Geometry: final body of the model. Coordinates: model frame, mm. A direction names the side the tool comes from. Give positions to 0.01 mm unless a question says otherwise; leave off trailing zeros. Write each loop counter-clockwise with the first axis right and the second up, starting at its lowest first coordinate (ties: lowest second). Pieces come first, ordered by that corner, then holes.
```python
from build123d import *

# Parameters (mm, degrees)
SKETCH001_W   = 70
SKETCH001_H   = 30
SKETCH001_R   = 3.9
SKETCH001_W_2 = 16
SKETCH001_H_2 = 17
PAD001_DEPTH  = 5
SKETCH002_W   = 70
SKETCH002_H   = 30
PAD002_DEPTH  = 5
SKETCH003_W   = 120
SKETCH003_H   = 30
PAD003_DEPTH  = 5
SKETCH004_W   = 120
SKETCH004_H   = 30
PAD004_DEPTH  = 5
SKETCH005_W   = 5
SKETCH005_H   = 5
SKETCH005_R   = 1
PAD005_DEPTH  = 30
SKETCH007_W   = 5
SKETCH007_H   = 5
SKETCH007_R   = 1
PAD006_DEPTH  = 30
SKETCH008_W   = 5
SKETCH008_H   = 5
SKETCH008_R   = 1
PAD007_DEPTH  = 30
SKETCH009_W   = 5
SKETCH009_H   = 5
SKETCH009_R   = 1
PAD008_DEPTH  = 30
SKETCH_R      = 2.5
PAD_DEPTH     = 5


with BuildPart() as body001:
    # Sketch001 → Pad001 (new body)
    with BuildSketch(Plane.XZ):
        with Locations((0, 15)):
            Rectangle(SKETCH001_W, SKETCH001_H)
        with Locations((-20, 15)):
            Circle(SKETCH001_R, mode=Mode.SUBTRACT)
        with Locations((8, 8.5)):
            Rectangle(SKETCH001_W_2, SKETCH001_H_2, mode=Mode.SUBTRACT)
    extrude(amount=PAD001_DEPTH)


with BuildPart() as body001_1:
    # Body001 placement: moved
    add(body001.part.moved(Location((0, -60, 0))))


with BuildPart() as body002:
    # Sketch002 → Pad002 (new body)
    with BuildSketch(Plane.XZ):
        with Locations((-105, 15)):
            Rectangle(SKETCH002_W, SKETCH002_H)
    extrude(amount=PAD002_DEPTH)


with BuildPart() as body002_1:
    # Body002 placement: moved
    add(body002.part.moved(Location((105, 65, 0))))


with BuildPart() as body003:
    # Sketch003 → Pad003 (new body)
    with BuildSketch(Plane.YZ):
        with Locations((0, 15)):
            Rectangle(SKETCH003_W, SKETCH003_H)
    extrude(amount=PAD003_DEPTH)


with BuildPart() as body003_1:
    # Body003 placement: moved
    add(body003.part.moved(Location((30, 0, 0))))


with BuildPart() as body004:
    # Sketch004 → Pad004 (new body)
    with BuildSketch(Plane.YZ):
        with Locations((0, 15)):
            Rectangle(SKETCH004_W, SKETCH004_H)
    extrude(amount=PAD004_DEPTH)


with BuildPart() as body004_1:
    # Body004 placement: moved
    add(body004.part.moved(Location((-35, 0, 0))))


with BuildPart() as hole_in_the_right_frame:
    # Sketch005 → Pad005 (new body)
    with BuildSketch(Plane.XY):
        with Locations((27.5, 42.5)):
            Rectangle(SKETCH005_W, SKETCH005_H)
        with Locations((27.5, 42.5)):
            Circle(SKETCH005_R, mode=Mode.SUBTRACT)
    extrude(amount=PAD005_DEPTH)


with BuildPart() as hole_in_the_right_frame_1:
    # Body005 placement: moved
    add(hole_in_the_right_frame.part.moved(Location((0, 15, 0))))


with BuildPart() as hole_in_the_left_frame:
    # Sketch007 → Pad006 (new body)
    with BuildSketch(Plane.XY):
        with Locations((-27.5, 42.5)):
            Rectangle(SKETCH007_W, SKETCH007_H)
        with Locations((-27.5, 42.5)):
            Circle(SKETCH007_R, mode=Mode.SUBTRACT)
    extrude(amount=PAD006_DEPTH)


with BuildPart() as hole_in_the_left_frame_1:
    # Body006 placement: moved
    add(hole_in_the_left_frame.part.moved(Location((0, 15, 0))))


with BuildPart() as hole_in_the_left_frame1:
    # Sketch008 → Pad007 (new body)
    with BuildSketch(Plane.XY):
        with Locations((-27.5, -42.5)):
            Rectangle(SKETCH008_W, SKETCH008_H)
        with Locations((-27.5, -42.5)):
            Circle(SKETCH008_R, mode=Mode.SUBTRACT)
    extrude(amount=PAD007_DEPTH)


with BuildPart() as hole_in_the_left_frame1_1:
    # Body007 placement: moved
    add(hole_in_the_left_frame1.part.moved(Location((0, -15, 0))))


with BuildPart() as body008:
    # Sketch009 → Pad008 (new body)
    with BuildSketch(Plane.XY):
        with Locations((27.5, -42.5)):
            Rectangle(SKETCH009_W, SKETCH009_H)
        with Locations((27.5, -42.5)):
            Circle(SKETCH009_R, mode=Mode.SUBTRACT)
    extrude(amount=PAD008_DEPTH)


with BuildPart() as body008_1:
    # Body008 placement: moved
    add(body008.part.moved(Location((0, -15, 0))))


with BuildPart() as fusion:
    # Sketch → Pad (new body)
    with BuildSketch(Plane.XY):
        with BuildLine():
            Line((-35.022389, 65), (35, 65))
            ThreePointArc((45, 55), (42.071068, 62.071068), (35, 65))
            Line((45, 55), (45, -55))
            ThreePointArc((35, -65), (42.071068, -62.071068), (45, -55))
            Line((35, -65), (-35, -65))
            ThreePointArc((-45, -55), (-42.071068, -62.071068), (-35, -65))
            Line((-45, -55), (-45, 55.022389))
            ThreePointArc((-35.022389, 65), (-42.077625, 62.077625), (-45, 55.022389))
        make_face()
        with Locations((40, -55)):
            Circle(SKETCH_R, mode=Mode.SUBTRACT)
        with Locations((40, 55)):
            Circle(SKETCH_R, mode=Mode.SUBTRACT)
        with Locations((-40, -55)):
            Circle(SKETCH_R, mode=Mode.SUBTRACT)
        with Locations((-40, 55)):
            Circle(SKETCH_R, mode=Mode.SUBTRACT)
    extrude(amount=PAD_DEPTH)

    # Fusion: union Body001, Body002, Body003, Body004, Hole in the right frame, Hole in the left frame, Hole in the left frame1, Body008
    add(body001_1.part)
    add(body002_1.part)
    add(body003_1.part)
    add(body004_1.part)
    add(hole_in_the_right_frame_1.part)
    add(hole_in_the_left_frame_1.part)
    add(hole_in_the_left_frame1_1.part)
    add(body008_1.part)


solid = fusion.part
```
Item 1: Section A-A, the plane z = 8. Return the cut outline in (x, y), plus the area to 3 significant figures.
Found:
outline: (-35, -65) - (0, -65) - (0, -60) - (-25, -60) - (-25, -55) - (-30, -55) - (-30, 55) - (-25, 55) - (-25, 60) - (25, 60) - (25, 55) - (30, 55) - (30, -55) - (25, -55) - (25, -60) - (16, -60) - (16, -65) - (35, -65) - (35, 65) - (-35, 65) - close; hole circle Ø2 at (-27.5, -57.5); hole circle Ø2 at (-27.5, 57.5); hole circle Ø2 at (27.5, -57.5); hole circle Ø2 at (27.5, 57.5)
area: 1,910 mm2
Item 2: Line query: L1, parallel to X at y = 57.5, z = 22.75; L2, parallel to X at y = 22.5, z = 24; L3, parallel to Y at x = 5.5, z = 28.25. Output: solid intervals per line, ascending.
Found:
L1: x = -35 to -28.5, -26.5 to -25, 25 to 26.5, 28.5 to 35
L2: x = -35 to -30, 30 to 35
L3: y = -65 to -60, 60 to 65
Item 3: Section D-D, the plane x = -40. Return the cut outline in (y, z).
Found:
outline: (-63.66, 0) - (-57.5, 0) - (-57.5, 5) - (-63.66, 5) - close; (-52.5, 0) - (52.5, 0) - (52.5, 5) - (-52.5, 5) - close; (57.5, 0) - (63.67, 0) - (63.67, 5) - (57.5, 5) - close
Item 4: Section B-B, the plane z = 15. Return the cut outline in (x, y), plus the area to 3 significant figures.
Found:
outline: (-35, -65) - (-23.9, -65) - (-23.9, -60) - (-25, -60) - (-25, -55) - (-30, -55) - (-30, 55) - (-25, 55) - (-25, 60) - (25, 60) - (25, 55) - (30, 55) - (30, -55) - (25, -55) - (25, -60) - (16, -60) - (16, -65) - (35, -65) - (35, 65) - (-35, 65) - close; (-16.1, -65) - (0, -65) - (0, -60) - (-16.1, -60) - close; hole circle Ø2 at (-27.5, -57.5); hole circle Ø2 at (-27.5, 57.5); hole circle Ø2 at (27.5, -57.5); hole circle Ø2 at (27.5, 57.5)
area: 1,870 mm2
Item 5: Pin query (flat end, axial travel): pin 1 Ø6 at (y, z) = (-39.5, 12.5) entering from +X; pin 2 Ø10 at (x, y) = (6.5, 20.5) entering from +Z; pin 3 Ø6 at (y, z) = (-12.5, 17) entering from -X. Return the tip coordinate at first contact, or that it passes through.
Found:
pin 1: stops at x = 35
pin 2: stops at z = 5
pin 3: stops at x = -35
Item 6: Reachability of faces 1 (the face through (-37.69, 54.04, 2.46)), 2 (the face through (27, 55, 17)), 3 (the face through (35, 1, 17)) from +Z, -Z, +X, -X, +Y, -Y: full face, straight path, thin tool, end or side. Return the list, or none.
Found:
face 1: +Z, -Z
face 2: +Z
face 3: +Z, +X, +Y, -Y
Item 7: Section C-C, the plane y = 26. Return the cut outline in (x, z).
Found:
outline: (-45, 0) - (45, 0) - (45, 5) - (35, 5) - (35, 30) - (30, 30) - (30, 5) - (-30, 5) - (-30, 30) - (-35, 30) - (-35, 5) - (-45, 5) - close
Item 8: Pull-direction query (Z, two-part tool) for faces 4 (the face through (-40, 1, 5)), 5 (the face through (-42.15, -61.99, 2.46)), 6 (the face through (16, -62, 11)), 7 (the face through (-1, 1, 0)); classes: +Z half, -Z half, draft (parallel to the pull), parting line (faces both ways), or undercut.
Found:
face 4: +Z half
face 5: draft
face 6: undercut
face 7: -Z half
